CAD build for the part. Positions are in the model's coordinates, mm. Round coordinates to 2 decimals unless told otherwise and drop trailing zeros. Loops run counter-clockwise (first coordinate to the right, second up) from the corner with the lowest first, then second, coordinate; pieces in that order, holes last.
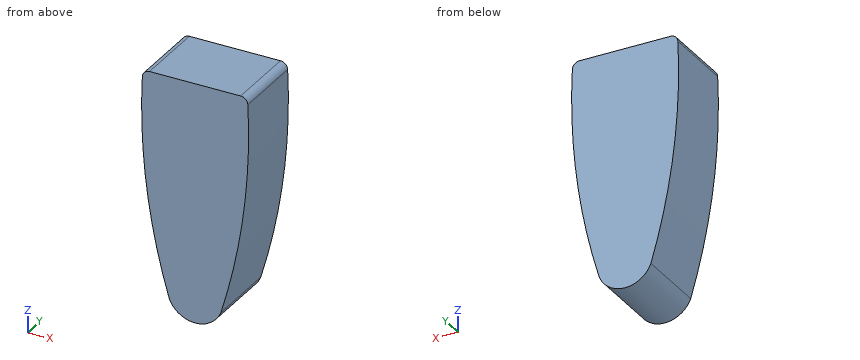
from build123d import *

# Parameters (mm, degrees)
F1_DEPTH = 100


with BuildPart() as f1:
    # F0 (on Front) → F1 (new body)
    with BuildSketch(Plane.XZ):
        with BuildLine():
            Line((66.602687, 55.139948), (-59.430013, 55.139948))
            ThreePointArc((-59.430013, 55.139948), (-66.330961, 52.377138), (-69.418707, 45.615332))
            ThreePointArc((-69.418707, 45.615332), (-63.634498, -105.241982), (-32.151404, -252.890894))
            ThreePointArc((-32.151404, -252.890894), (3.586337, -277.094579), (39.324078, -252.890894))
            ThreePointArc((39.324078, -252.890894), (70.807172, -105.241982), (76.591381, 45.615332))
            ThreePointArc((76.591381, 45.615332), (73.503635, 52.377138), (66.602687, 55.139948))
        make_face()
    extrude(amount=F1_DEPTH)


solid = f1.part
Item 1: Cut at A-A (y = -41.5). List the corners of the cut face in (x, z).
Verdict:
outline: (-69.42, 45.62) arc R880.03 ccw to (-32.15, -252.89) arc R38.49 ccw to (39.32, -252.89) arc R880.03 ccw to (76.59, 45.62) arc R10 ccw to (66.6, 55.14) - (-59.43, 55.14) arc R10 ccw to start
Item 2: Cut at C-C (x = 52). List the corners of the cut face in (y, z).
Verdict:
outline: (-100, -206.88) - (0, -206.88) - (0, 55.14) - (-100, 55.14) - close
Item 3: Flat gauge pins, fed straight in: P1, Ø6, axis at x = -12, y = -36.5, coming from the -Z side; P2, Ø2, axis at x = -7.5, y = -25, coming from the -Z side; P3, Ø6, axis at y = -19, z = -224, coming from the -X side. Where does each tip first touch, or does it go through?
Verdict:
P1: stops at z = -274.98
P2: stops at z = -275.75
P3: stops at x = -41.22
Item 4: Wall check: L1, parallel to X at y = -36, z = -28; L2, parallel to X at y = -54.5, z = -139.5; L3, parallel to Z at x = 21.5, y = -67.5. Give the ranges that are in metal, low to high.
Verdict:
L1: x = -69.84 to 77.01
L2: x = -58.67 to 65.84
L3: z = -272.67 to 55.14
Item 5: Cut at B-B (z = -155). List the corners of the cut face in (x, y), plus the area to 3 significant figures.
Verdict:
outline: (-55.97, -100) - (63.14, -100) - (63.14, 0) - (-55.97, 0) - close
area: 11,900 mm2
